Can you work these out from the model? Positions are in its coordinate system, mm. Give positions to 0.01 mm unless a question says otherwise; leave off trailing zeros. Order: outer loops, then holes, each group sorted by start corner. A loop starts at its lowest first (then second) coordinate and runs counter-clockwise, first axis right, second up. Notation, with made-up numbers: (87.25, 22) - (129.25, 22) arc R17 cw to (129.25, 49) - close; hole circle Ø2 at (10.5, -13.75). An arc over 180 degrees is marked (long way). Answer as a JSON object with one key per item and string values.
```python
from build123d import *

# Parameters (mm, degrees)
CROQUIS1_W              = 160
CROQUIS1_H              = 160
CROQUIS1_R              = 1.5
CROQUIS1_R_2            = 2.5
CROQUIS1_W_2            = 39
CROQUIS1_H_2            = 120
CROQUIS1_W_3            = 30
CROQUIS1_W_4            = 5
CROQUIS1_H_3            = 7
CROQUIS1_W_5            = 7
CROQUIS1_H_4            = 5
SALIENTE_EXTRUIR1_DEPTH = 2
CROQUIS2_W              = 160
CROQUIS2_H              = 160
CORTAR_EXTRUIR1_DEPTH   = 10


with BuildPart() as part:
    # Croquis1 → Saliente-Extruir1 (new body)
    with BuildSketch(Plane(origin=(0, 0, 0), x_dir=(1, 0, 0), z_dir=(0, 1, 0))):
        with Locations((70, 70)):
            Rectangle(CROQUIS1_W, CROQUIS1_H)
        with Locations(Location((52, 81.25, 0), (0, 0, 270))):
            Circle(CROQUIS1_R, mode=Mode.SUBTRACT)
        with Locations(Location((52, 58.75, 0), (0, 0, 270))):
            Circle(CROQUIS1_R, mode=Mode.SUBTRACT)
        with Locations(Location((0, 140, 0), (0, 0, 270))):
            Circle(CROQUIS1_R_2, mode=Mode.SUBTRACT)
        with Locations(Location((0, 0, 0), (0, 0, 270))):
            Circle(CROQUIS1_R_2, mode=Mode.SUBTRACT)
        with Locations(Location((88, 81.25, 0), (0, 0, 90))):
            Circle(CROQUIS1_R, mode=Mode.SUBTRACT)
        with Locations(Location((88, 58.75, 0), (0, 0, 90))):
            Circle(CROQUIS1_R, mode=Mode.SUBTRACT)
        with Locations(Location((140, 0, 0), (0, 0, 90))):
            Circle(CROQUIS1_R_2, mode=Mode.SUBTRACT)
        with Locations(Location((140, 140, 0), (0, 0, 90))):
            Circle(CROQUIS1_R_2, mode=Mode.SUBTRACT)
        with Locations((29.5, 70)):
            Rectangle(CROQUIS1_W_2, CROQUIS1_H_2, mode=Mode.SUBTRACT)
        with Locations((110.5, 70)):
            Rectangle(CROQUIS1_W_2, CROQUIS1_H_2, mode=Mode.SUBTRACT)
        with Locations((70, 70)):
            Rectangle(CROQUIS1_W_3, CROQUIS1_H_2, mode=Mode.SUBTRACT)
        with Locations((140, 70)):
            Rectangle(CROQUIS1_W_4, CROQUIS1_H_3, mode=Mode.SUBTRACT)
        with Locations((70, 140)):
            Rectangle(CROQUIS1_W_5, CROQUIS1_H_4, mode=Mode.SUBTRACT)
    extrude(amount=SALIENTE_EXTRUIR1_DEPTH)

    # Croquis2 → Cortar-Extruir1 (cut)
    with BuildSketch(Plane(origin=(0, 2, 0), x_dir=(1, 0, 0), z_dir=(0, 1, 0))):
        with Locations((70, 70)):
            Rectangle(CROQUIS2_W, CROQUIS2_H)
        with BuildLine():
            Line((0, 147.5), (140, 147.5))
            ThreePointArc((140, 147.5), (145.303300859, 145.303300859), (147.5, 140))
            Line((147.5, 140), (147.5, 0))
            ThreePointArc((147.5, 0), (145.303300859, -5.303300859), (140, -7.5))
            Line((140, -7.5), (0, -7.5))
            ThreePointArc((0, -7.5), (-5.303300859, -5.303300859), (-7.5, 0))
            Line((-7.5, 0), (-7.5, 140))
            ThreePointArc((-7.5, 140), (-5.303300859, 145.303300859), (0, 147.5))
        make_face(mode=Mode.SUBTRACT)
    extrude(amount=-CORTAR_EXTRUIR1_DEPTH, mode=Mode.SUBTRACT)


solid = part.part
```
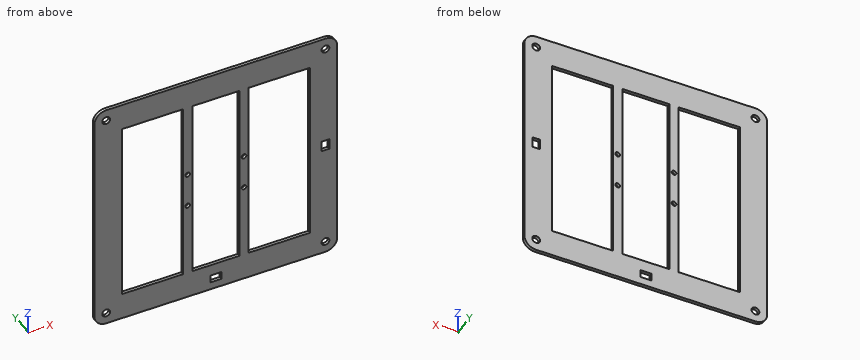
Q1. I need wall thicknesses on L1, parallel to X at y = 1.6, z = -81.25; L2, parallel to X at y = 0.3, z = -69; L3, parallel to Z at x = 88, y = 0.6. Which ranges of each line are inside material? Lowest first, please.
Recorded:
{"L1": "x = -7.5 to 10, 49 to 50.5, 53.5 to 55, 85 to 86.5, 89.5 to 91, 130 to 147.5", "L2": "x = -7.5 to 10, 49 to 55, 85 to 91, 130 to 137.5, 142.5 to 147.5", "L3": "z = -147.5 to -82.75, -79.75 to -60.25, -57.25 to 7.5"}
Q2. If we section it at A-A, the plane z = -88: Please give me the cut outline in (x, y).
Recorded:
{"outline": "(-7.5, 0) - (10, 0) - (10, 2) - (-7.5, 2) - close; (49, 0) - (55, 0) - (55, 2) - (49, 2) - close; (85, 0) - (91, 0) - (91, 2) - (85, 2) - close; (130, 0) - (147.5, 0) - (147.5, 2) - (130, 2) - close"}
Q3. If we section it at C-C, the plane y = 0.8: Count the separate pieces of the cut face and the enclosed holes in it, then the cut area to 3 significant figures.
Recorded:
{"separate pieces": "1", "enclosed holes": "13", "area": "10,800 mm^2"}
Q4. I'm going to push a flat-ended pin straight in: pin 1 Ø2.5 at (x, z) = (88, -58.75) entering from +Y. Where does the tip first touch, or does it pass through?
Recorded:
{"pin 1": "passes through"}
Q5. If we section it at B-B, the plane z = -70: Please give me the cut outline in (x, y), then the cut area to 3 significant figures.
Recorded:
{"outline": "(-7.5, 0) - (10, 0) - (10, 2) - (-7.5, 2) - close; (49, 0) - (55, 0) - (55, 2) - (49, 2) - close; (85, 0) - (91, 0) - (91, 2) - (85, 2) - close; (130, 0) - (137.5, 0) - (137.5, 2) - (130, 2) - close; (142.5, 0) - (147.5, 0) - (147.5, 2) - (142.5, 2) - close", "area": "84.0 mm^2"}
